from build123d import *

# Parameters (mm, degrees)
SKETCH2_W           = 63.5
SKETCH2_H           = 63.5
BOSS_EXTRUDE1_DEPTH = 5
SKETCH3_R           = 2.2
SKETCH3_W           = 21.25
SKETCH3_H           = 41.25
CUT_EXTRUDE1_DEPTH  = 6


with BuildPart() as part:
    # Sketch2 → Boss-Extrude1 (new body)
    with BuildSketch(Plane(origin=(0, 0, 0), x_dir=(1, 0, 0), z_dir=(0, 1, 0))):
        Rectangle(SKETCH2_W, SKETCH2_H)
    extrude(amount=BOSS_EXTRUDE1_DEPTH)

    # Sketch3 → Cut-Extrude1 (cut, through all)
    with BuildSketch(Plane(origin=(0, 5, 0), x_dir=(1, 0, 0), z_dir=(0, 1, 0))):
        with Locations((5.325, 24.725)):
            Circle(SKETCH3_R)
        with Locations((-5.325, 24.725)):
            Circle(SKETCH3_R)
        with Locations((5.325, -24.725)):
            Circle(SKETCH3_R)
        with Locations((-5.325, -24.725)):
            Circle(SKETCH3_R)
        Rectangle(SKETCH3_W, SKETCH3_H)
    extrude(amount=-CUT_EXTRUDE1_DEPTH, mode=Mode.SUBTRACT)


solid = part.part
Read the model definition and answer for the solid it produces. Units are mm, in the model's axes. A direction names the side the tool comes from. Give positions to 0.01 mm unless a question says otherwise; leave off trailing zeros. Write each loop counter-clockwise with the first axis right and the second up, starting at its lowest first coordinate (ties: lowest second). Pieces come first, ordered by that corner, then holes. Notation, with made-up numbers: (-33, -31.5) -> (23, -31.5) arc R22 ccw to (23, -6.5) -> close; hole circle Ø7 at (27, 22.5). An arc over 180 degrees is marked (long way). Answer as a JSON object with one key per item and string values. Group by question number.
1) A tool of negligible diameter and unlimited length cuts with its end or side. For faces 1 (the flat face through (10.625, 3, 0)), 2 (the flat face through (14, 5, 0)), from which of +Z, -Z, +X, -X, +Y, -Y can it reach the whole face along a straight path? Write none if from no direction.
2) Consider L1, parallel to Z at x = -10, y = 4.45 (3 decimals); L2, parallel to X at y = 1, z = -5 (3 decimals); L3, parallel to Z at x = 6, y = 1.25 (3 decimals). Determine where each line is inside the solid, lowest interval first. Write a range as from..to.
3) Find section A-A (z = 8). Write down the section's boundary in (x, y) (3 decimals).
4) The mould has two halves that part along Z. Classify faces 3 (the flat face through (14, 0, 0)), 4 (the flat face through (0, 3, 20.625)), 5 (the flat face through (0, 2, -31.75)), 6 (the flat face through (-10.625, 3, 0)): +Z half, -Z half, draft (parallel to the pull), parting line (faces both ways), or undercut.
5) Find section B-B (y = 3.6). Write down the section's boundary in (x, z) (3 decimals).
Values follow:
{
 "1": {"face 1": "+Y, -Y", "face 2": "+Z, -Z, +X, -X, +Y"},
 "2": {"L1": "z = -31.75..-20.625, 20.625..31.75", "L2": "x = -31.75..-10.625, 10.625..31.75", "L3": "z = -31.75..-26.819, -22.631..-20.625, 20.625..22.631, 26.819..31.75"},
 "3": {"outline": "(-31.75, 0) -> (-10.625, 0) -> (-10.625, 5) -> (-31.75, 5) -> close; (10.625, 0) -> (31.75, 0) -> (31.75, 5) -> (10.625, 5) -> close"},
 "4": {"face 3": "draft", "face 4": "undercut", "face 5": "-Z half", "face 6": "undercut"},
 "5": {"outline": "(-31.75, -31.75) -> (31.75, -31.75) -> (31.75, 31.75) -> (-31.75, 31.75) -> close; hole (-10.625, -20.625) -> (10.625, -20.625) -> (10.625, 20.625) -> (-10.625, 20.625) -> close; hole circle Ø4.4 at (-5.325, -24.725); hole circle Ø4.4 at (-5.325, 24.725); hole circle Ø4.4 at (5.325, -24.725); hole circle Ø4.4 at (5.325, 24.725)"}
}
